Answer from the drawing. Dimensions are ordinates in mm from the lowest x, y and z of the part. Give positions to 0.01 mm unless a question says otherwise; leave off trailing zeros. Write each loop counter-clockwise with the first axis right and the second up, starting at its lowest first coordinate (ties: lowest second). Pieces come first, ordered by that corner, then holes.
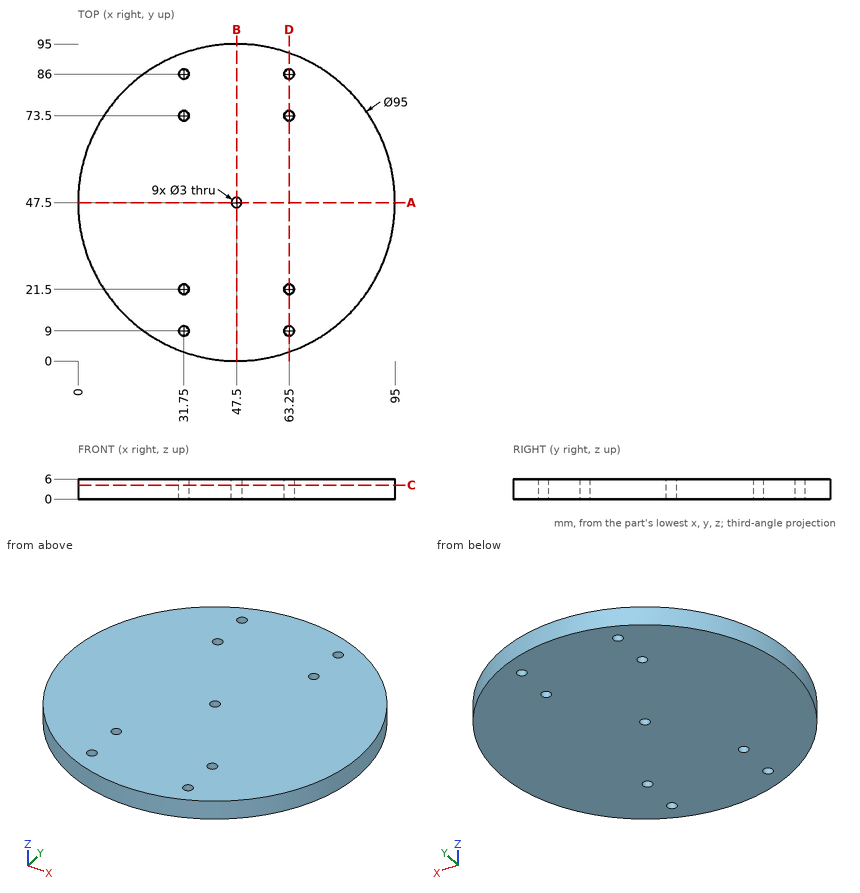
Item 1: Each of these flat-tipped pins is pushed along its axis until it touches: P1, Ø3, axis at y = 71, z = 4.5, coming from the -X side; P2, Ø3, axis at x = 30, z = 5, coming from the +Y side; P3, Ø1, axis at x = 62, z = 5, coming from the +Y side. Where does it stop, or does it pass through?
Conclusion:
P1: stops at x = 5.4
P2: stops at y = 92.22
P3: stops at y = 92.89
Item 2: A cutting plane is placed at D-D, the plane x = 63.25. Give the vertices of the cut face in (y, z), plus the area to 3 significant figures.
Conclusion:
outline: (2.69, 0) - (7.5, 0) - (7.5, 6) - (2.69, 6) - close; (10.5, 0) - (20, 0) - (20, 6) - (10.5, 6) - close; (23, 0) - (72, 0) - (72, 6) - (23, 6) - close; (75, 0) - (84.5, 0) - (84.5, 6) - (75, 6) - close; (87.5, 0) - (92.31, 0) - (92.31, 6) - (87.5, 6) - close
area: 466 mm2
Item 3: A cutting plane is placed at A-A, the plane y = 47.5. Give the vertices of the cut face in (x, z), plus the area to 3 significant figures.
Conclusion:
outline: (0, 0) - (46, 0) - (46, 6) - (0, 6) - close; (49, 0) - (95, 0) - (95, 6) - (49, 6) - close
area: 552 mm2
Item 4: A cutting plane is placed at C-C, the plane z = 4.15. Count the separate pieces of the cut face and the enclosed holes in it, plus the area to 3 significant figures.
Conclusion:
separate pieces: 1
enclosed holes: 9
area: 7,020 mm2
Item 5: Consider probe 1 along Y at (x, z) = (31.75, 3.65); probe 2 along X at (y, z) = (8.5, 0.85); probe 3 along X at (y, z) = (86, 4.45). Determine where each line is inside the solid, lowest interval first.
Conclusion:
probe 1: y = 2.69 to 7.5, 10.5 to 20, 23 to 72, 75 to 84.5, 87.5 to 92.31
probe 2: x = 20.38 to 30.34, 33.16 to 61.84, 64.66 to 74.62
probe 3: x = 19.68 to 30.25, 33.25 to 61.75, 64.75 to 75.32
